The model under review builds one solid part; all positions refer to its coordinate system, in mm. Face numbers are marked on the shaded views. A direction names the side the tool comes from. Round coordinates to 2 decimals unless told otherwise and drop trailing zeros. Loops run counter-clockwise (first coordinate to the right, second up) from the corner with the lowest first, then second, coordinate; pieces in that order, holes last. Notation, with made-up numbers: (35, -9) -> (56, -9) arc R33 ccw to (56, 25) -> close; hole circle Ø3 at (-7.75, 80.5). An arc over 180 degrees is marked (long way). Use CSV: the item, a comma, the result in double quotes. Start each with the question number.
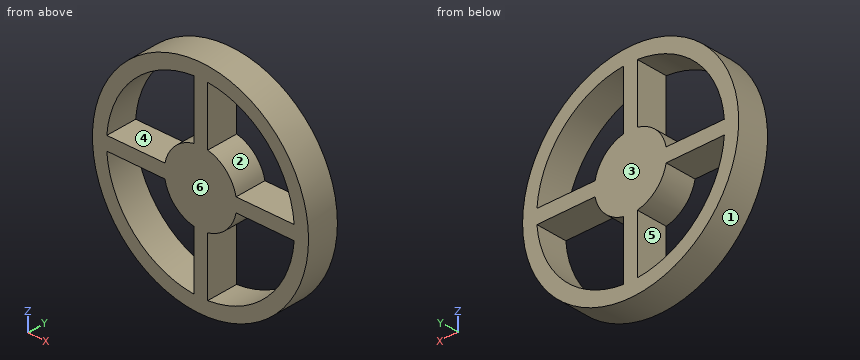
```python
from build123d import *

# Parameters (mm, degrees)
F0_R     = 10.954504
F1_DEPTH = 3.175


with BuildPart() as f1:
    # F0 (on Front) → F1 (new body)
    with BuildSketch(Plane.XZ):
        Circle(F0_R)
        with BuildLine():
            ThreePointArc((9.499057, 0.702522), (9.518512, 0.3515), (9.525, 0))
            ThreePointArc((9.525, 0), (9.518348, -0.355918), (9.498401, -0.711339))
            ThreePointArc((9.498401, -0.711339), (6.742333, -6.728043), (0.73149, -9.49687))
            ThreePointArc((0.73149, -9.49687), (0.026314, -9.524964), (-0.679006, -9.500767))
            ThreePointArc((-0.679006, -9.500767), (-6.739803, -6.730578), (-9.501688, -0.665992))
            ThreePointArc((-9.501688, -0.665992), (-9.524982, 0.018312), (-9.499057, 0.702522))
            ThreePointArc((-9.499057, 0.702522), (-6.726851, 6.743523), (-0.679006, 9.500767))
            ThreePointArc((-0.679006, 9.500767), (0.026314, 9.524964), (0.73149, 9.49687))
            ThreePointArc((0.73149, 9.49687), (6.745455, 6.724913), (9.499057, 0.702522))
        make_face(mode=Mode.SUBTRACT)
        with BuildLine():
            ThreePointArc((3.668611, 0), (3.651599, 0.352898), (3.600718, 0.702522))
            ThreePointArc((3.600718, 0.702522), (2.604522, 2.583636), (0.73149, 3.594945))
            ThreePointArc((0.73149, 3.594945), (0.026741, 3.668514), (-0.679006, 3.605227))
            ThreePointArc((-0.679006, 3.605227), (-2.58562, 2.602552), (-3.600718, 0.702522))
            ThreePointArc((-3.600718, 0.702522), (-3.668605, 0.007053), (-3.603393, -0.688672))
            ThreePointArc((-3.603393, -0.688672), (-2.590619, -2.597576), (-0.679006, -3.605227))
            ThreePointArc((-0.679006, -3.605227), (0.026741, -3.668514), (0.73149, -3.594945))
            ThreePointArc((0.73149, -3.594945), (2.609484, -2.578624), (3.603393, -0.688672))
            ThreePointArc((3.603393, -0.688672), (3.65227, -0.345877), (3.668611, 0))
        make_face()
        with BuildLine():
            ThreePointArc((-0.679006, -9.500767), (0.026314, -9.524964), (0.73149, -9.49687))
            Line((0.73149, -9.49687), (0.73149, -3.594945))
            ThreePointArc((0.73149, -3.594945), (0.026741, -3.668514), (-0.679006, -3.605227))
            Line((-0.679006, -3.605227), (-0.679006, -9.500767))
        make_face()
        with BuildLine():
            Line((-3.600718, 0.702522), (-9.499057, 0.702522))
            ThreePointArc((-9.499057, 0.702522), (-9.524982, 0.018312), (-9.501688, -0.665992))
            Line((-9.501688, -0.665992), (-3.603393, -0.688672))
            ThreePointArc((-3.603393, -0.688672), (-3.668605, 0.007053), (-3.600718, 0.702522))
        make_face()
        with BuildLine():
            ThreePointArc((9.498401, -0.711339), (9.518348, -0.355918), (9.525, 0))
            ThreePointArc((9.525, 0), (9.518512, 0.3515), (9.499057, 0.702522))
            Line((9.499057, 0.702522), (3.600718, 0.702522))
            ThreePointArc((3.600718, 0.702522), (3.651599, 0.352898), (3.668611, 0))
            ThreePointArc((3.668611, 0), (3.65227, -0.345877), (3.603393, -0.688672))
            Line((3.603393, -0.688672), (9.498401, -0.711339))
        make_face()
        with BuildLine():
            Line((0.73149, 3.594945), (0.73149, 9.49687))
            ThreePointArc((0.73149, 9.49687), (0.026314, 9.524964), (-0.679006, 9.500767))
            Line((-0.679006, 9.500767), (-0.679006, 3.605227))
            ThreePointArc((-0.679006, 3.605227), (0.026741, 3.668514), (0.73149, 3.594945))
        make_face()
    extrude(amount=F1_DEPTH)


solid = f1.part
```
1. Clearance check with flat-ended pins moving along their axes: P1, Ø1, axis at y = -2, z = 7.5, coming from the +X side; P2, Ø1.6, axis at y = -1.5, z = 6.5, coming from the -X side; P3, Ø1.6, axis at x = 6.5, y = -1, coming from the +Z side; P4, Ø10, axis at x = -4, z = 3, coming from the +Y side. State where each tip first meets the part, or that it passes through.
2. For line 1 along X through (y, z) = (-0.3, -2.25); line 2 along X through (y, z) = (-0.2, 4.25); line 3 along Z through (x, y) = (-3, -0.45), list the stretches that pass through material, from the lowest coordinate up. Write a range as from..to.
3. The part is to be moulded in two halves that separate along X. For the marked faces 1, 2, 3 and 4, say which applies: pulls with the +X half, pulls with the -X half, needs draft (parallel to the pull), parting line crosses it, or undercut.
4. Take a section at A-A, the plane y = -0.7. Count the separate pieces of the cut face and the enclosed holes in it, then the cut area to 3 significant figures.
5. For the marked faces 5 and 6, list the 3-axis set-ups (+Z, -Z, +X, -X, +Y, -Y) from which the entire face can be reached by the end or side of a thin tool; tool diameter is ignored.
6. Take a section at C-C, the plane z = 7.5. Give the boundary of the cut face in (x, y) (1 decimal).
7. Take a section at B-B, the plane x = 8.5. Give the boundary of the cut face in (y, z) (1 decimal).
Results:
1,P1,"x = 8.43"
1,P2,"x = -9.35"
1,P3,"z = 9.35"
1,P4,"y = 0"
2,line 1,"-10.72..-9.26, -2.9..2.9, 9.26..10.72"
2,line 2,"-10.1..-8.52, -0.68..0.73, 8.52..10.1"
2,line 3,"-10.54..-9.04, -2.11..2.11, 9.04..10.54"
3,face 1,"parting line crosses it"
3,face 2,"undercut"
3,face 3,"needs draft"
3,face 4,"undercut"
4,separate pieces,"1"
4,enclosed holes,"4"
4,area,"167 mm²"
5,face 5,"+Y, -Y"
5,face 6,"+Z, -Z, +X, -X, -Y"
6,outline,"(-8, -3.2) -> (-5.9, -3.2) -> (-5.9, 0) -> (-8, 0) -> close; (-0.7, -3.2) -> (0.7, -3.2) -> (0.7, 0) -> (-0.7, 0) -> close; (5.9, -3.2) -> (8, -3.2) -> (8, 0) -> (5.9, 0) -> close"
7,outline,"(-3.2, -6.9) -> (0, -6.9) -> (0, -4.3) -> (-3.2, -4.3) -> close; (-3.2, -0.7) -> (0, -0.7) -> (0, 0.7) -> (-3.2, 0.7) -> close; (-3.2, 4.3) -> (0, 4.3) -> (0, 6.9) -> (-3.2, 6.9) -> close"
